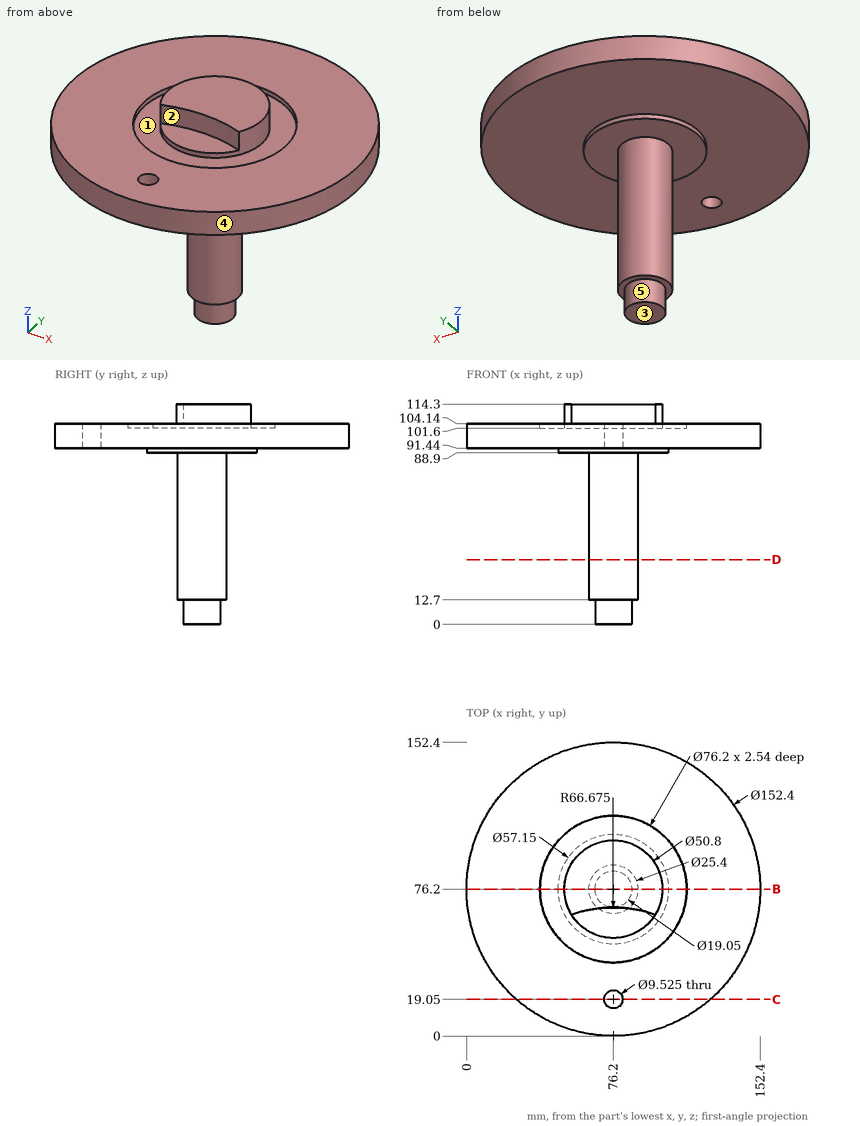
Source: three-view drawing plus pictorial views. Frame: mm from the lowest corner of the part. A direction names the side the tool comes from. Round coordinates to 2 decimals unless told otherwise and drop trailing zeros. Write each loop counter-clockwise with the first axis right and the second up, starting at its lowest first coordinate (ties: lowest second). Pieces come first, ordered by that corner, then holes. Notation, with made-up numbers: (46, 66) -> (51, 66) arc R36 cw to (51, 102) -> close; hole circle Ø5 at (40.5, 22). An arc over 180 degrees is marked (long way). Return JSON: item names as keys, results as strings.
Q1. Section C-C on y = 19.05. Return the cut outline in (x, z), and give its area (3 significant figures).
From the geometry:
{"outline": "(25.8, 91.44) -> (71.44, 91.44) -> (71.44, 104.14) -> (25.8, 104.14) -> close; (80.96, 91.44) -> (126.6, 91.44) -> (126.6, 104.14) -> (80.96, 104.14) -> close", "area": "1,160 mm2"}
Q2. Ray query, line 1 (Y direction, x = 76.2, z = 102.5); line 2 (Y direction, x = 76, z = 99); line 3 (Z direction, x = 66.5, y = 138). Return the intervals inside material, ascending.
From the geometry:
{"line 1": "0 to 14.29, 23.81 to 38.1, 50.8 to 101.6, 114.3 to 152.4", "line 2": "0 to 14.29, 23.81 to 152.4", "line 3": "91.44 to 104.14"}
Q3. Set-up query: the marked faces 1, 2, 3, 4 and 5. Return all of +Z, -Z, +X, -X, +Y, -Y with unobstructed straight access to the full face (end or side cutting, diameter ignored); none if empty.
From the geometry:
{"face 1": "+Z", "face 2": "+Z, -Y", "face 3": "-Z, +X, -X, +Y, -Y", "face 4": "+Z, -Z", "face 5": "-Z"}
Q4. Section D-D on z = 33.5. Return the cut outline in (x, y), and give its area (3 significant figures).
From the geometry:
{"outline": "circle Ø25.4 at (76.2, 76.2)", "area": "507 mm2"}
Q5. First-contact query: pin 1 Ø3 at (y, z) = (109.5, 94.5) entering from +X; pin 2 Ø5 at (x, y) = (16.5, 98) entering from +Z; pin 3 Ø3 at (x, y) = (97, 117) entering from -Z. Flat tips, straight axial feed; report the tip coordinate or a pass-through.
From the geometry:
{"pin 1": "x = 145.45", "pin 2": "z = 104.14", "pin 3": "z = 91.44"}
Q6. Section B-B on y = 76.2. Return the cut outline in (x, z) (3 decimals), and give its area (3 significant figures).
From the geometry:
{"outline": "(0, 91.44) -> (47.625, 91.44) -> (47.625, 88.9) -> (63.5, 88.9) -> (63.5, 12.7) -> (66.675, 12.7) -> (66.675, 0) -> (85.725, 0) -> (85.725, 12.7) -> (88.9, 12.7) -> (88.9, 88.9) -> (104.775, 88.9) -> (104.775, 91.44) -> (152.4, 91.44) -> (152.4, 104.14) -> (114.3, 104.14) -> (114.3, 101.6) -> (101.6, 101.6) -> (101.6, 114.3) -> (50.8, 114.3) -> (50.8, 101.6) -> (38.1, 101.6) -> (38.1, 104.14) -> (0, 104.14) -> close", "area": "4,710 mm2"}
